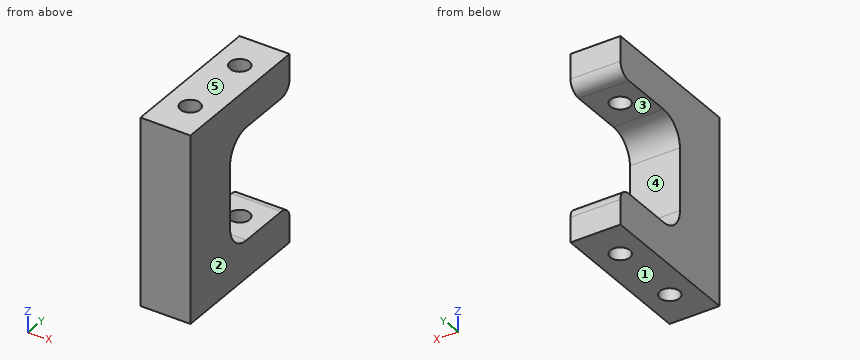
from build123d import *

# Parameters (mm, degrees)
SKETCH1_W                      = 6.35
SKETCH1_H                      = 19.05
BOSS_EXTRUDE2_DEPTH            = 23.8125
SKETCH2_W                      = 14.2875
SKETCH2_H                      = 11.43
WHEEL_SLOT_DEPTH               = 27.421265701
M3X0_5_TAPPED_HOLE1_AT_2_COUNT = 2
M3X0_5_TAPPED_HOLE1_AT_2_PITCH = 9.525
FILLET1_R                      = 3.175
FILLET2_R                      = 1.5875


with BuildPart() as part:
    # Sketch1 → Boss-Extrude2 (new body)
    with BuildSketch(Plane.XY):
        Rectangle(SKETCH1_W, SKETCH1_H)
    extrude(amount=BOSS_EXTRUDE2_DEPTH)

    # Sketch2 → WHEEL-SLOT (cut, through all)
    with BuildSketch(Plane(origin=(3.175, 0, 0), x_dir=(0, 0, -1), z_dir=(1, 0, 0))):
        with Locations((-11.90625, 3.81)):
            Rectangle(SKETCH2_W, SKETCH2_H)
    extrude(amount=-WHEEL_SLOT_DEPTH, mode=Mode.SUBTRACT)

    # Sketch4 → M3x0.5 Tapped Hole1 (revolve, cut)
    with BuildSketch(Plane(origin=(0, -4.7625, 23.8125), x_dir=(0, -1, 0), z_dir=(1, 0, 0))):
        Polygon((0, 0), (0, 10.657075774), (1.25, 9.906), (1.25, 0), align=None)
    m3x0_5_tapped_hole1 = revolve(axis=Axis((0, -4.7625, 30.1625), (0, 0, -1)), mode=Mode.SUBTRACT)

    # M3x0.5 Tapped Hole1 at 2: M3x0.5 Tapped Hole1 ×2
    with Locations(*[(0, i * M3X0_5_TAPPED_HOLE1_AT_2_PITCH, 0) for i in range(1, M3X0_5_TAPPED_HOLE1_AT_2_COUNT)]):
        add(m3x0_5_tapped_hole1, mode=Mode.SUBTRACT)

    # M3-TAPPED-MIR: M3x0.5 Tapped Hole1 across plane
    add(m3x0_5_tapped_hole1.mirror(Plane.XY.offset(11.90625)), mode=Mode.SUBTRACT)

    # M3-TAPPED-MIR copy 1 sketch → M3-TAPPED-MIR copy 1 (revolve, cut)
    with BuildSketch(Plane(origin=(0, 4.7625, 0), x_dir=(0, -1, 0), z_dir=(1, 0, 0))):
        Polygon((0, 0), (0, -10.657075774), (1.25, -9.906), (1.25, 0), align=None)
    revolve(axis=Axis((0, 4.7625, -6.35), (0, 0, -1)), mode=Mode.SUBTRACT)

    # Fillet1
    fillet1_edges = [part.edges().sort_by_distance(p)[0] for p in [
        (0, -1.905, 19.05),
        (0, -1.905, 4.7625),
    ]]
    fillet(fillet1_edges, radius=FILLET1_R)

    # Fillet2
    fillet2_edges = [part.edges().sort_by_distance(p)[0] for p in [
        (0, 9.525, 19.05),
        (0, 9.525, 4.7625),
    ]]
    fillet(fillet2_edges, radius=FILLET2_R)


solid = part.part
Geometry check sheet. Reference: the model listing, model coordinates, mm. Face numbers are marked on the shaded views. A direction names the side the tool comes from. Give positions to 0.01 mm unless a question says otherwise; leave off trailing zeros. Write each loop counter-clockwise with the first axis right and the second up, starting at its lowest first coordinate (ties: lowest second). Pieces come first, ordered by that corner, then holes. Notation, with made-up numbers: M 89.5,83 L 110.5,83 A32 ccw 110.5,119 Z; hole C -13,65.25 d9. An arc over 180 degrees is marked long. Answer as CSV lines item,"result". Start each with the question number.
Q1. Go/stop test with flat-tipped pins: pin 1 (1.5 mm diameter, centred on x = 0, z = 11, fed in from +Y) (3 decimals); pin 2 (5 mm diameter, centred on y = 6.5, z = 9, fed in from -X). Record where each tip stops, or that it passes through.
Q2. Release check for a two-part mould opening along Z. For the marked faces 1, 2 and 3 record: pulls with the +Z half, pulls with the -Z half, needs draft (parallel to the pull), parting line crosses it, or undercut.
Q3. Section check D-D, the plane z = 12. Record the cut outline in (x, y) (3 decimals), then the cut area to 3 significant figures.
Q4. Section check C-C, the plane z = 2.5. Give the number of separate pieces and of enclosed holes in the cut face, then the cut area to 3 significant figures.
Q5. Material ranges on L1, parallel to Z at x = -1.25, y = 5.25; L2, parallel to Y at x = 1, z = 20 (1 decimal); L3, parallel to Y at x = 1, z = 1 (1 decimal), recorded low to high.
Q6. Tool access check on the marked faces 4 and 5. Record the directions out of +Z, -Z, +X, -X, +Y, -Y that give a thin tool (end or side, any length) a straight path to the whole face; none if there is none.
Geometry says:
1,pin 1,"y = -1.905"
1,pin 2,"through"
2,face 1,"pulls with the -Z half"
2,face 2,"needs draft"
2,face 3,"undercut"
3,outline,"M -3.175,-9.525 L 3.175,-9.525 L 3.175,-1.905 L -3.175,-1.905 Z"
3,area,"48.4 mm^2"
4,separate pieces,"1"
4,enclosed holes,"2"
4,area,"111 mm^2"
5,L1,"0 to 4.76, 19.05 to 23.81"
5,L2,"-9.5 to -5.5, -4 to 4, 5.5 to 9.4"
5,L3,"-9.5 to -5.5, -4 to 4, 5.5 to 9.5"
6,face 4,"+X, -X, +Y"
6,face 5,"+Z, +X, -X, +Y, -Y"
